```python
from build123d import *

# Parameters (mm, degrees)
F0_W     = 152.4
F0_H     = 101.6
F1_DEPTH = 7.62
F2_T     = -2.54
F3_R     = 5.08


with BuildPart() as f1:
    # F0 (on Front) → F1 (new body)
    with BuildSketch(Plane.XZ):
        Rectangle(F0_W, F0_H)
    extrude(amount=F1_DEPTH)

    # F2
    f2_openings = [f1.faces().sort_by_distance(p)[0] for p in [
        (0, -7.62, 0),
    ]]
    offset(amount=F2_T, openings=f2_openings)

    # F3
    f3_edges = [f1.edges().sort_by_distance(p)[0] for p in [
        (-73.66, -5.08, 48.26),
        (-73.66, -5.08, -48.26),
        (73.66, -5.08, 48.26),
        (73.66, -5.08, -48.26),
    ]]
    fillet(f3_edges, radius=F3_R)


solid = f1.part
```
Read the model definition and answer for the solid it produces. Units are mm, in the model's axes. A direction names the side the tool comes from. Coordinates: 2 decimals unless noted, no trailing zeros. Loops run counter-clockwise (first coordinate to the right, second up) from the corner with the lowest first, then second, coordinate; pieces in that order, holes last.
(1) The part is cut by section B-B (x = 49). Determine the outline of the cut face in (y, z), and give its area (3 significant figures).
Solution:
outline: (-7.62, -50.8) - (0, -50.8) - (0, 50.8) - (-7.62, 50.8) - (-7.62, 48.26) - (-2.54, 48.26) - (-2.54, -48.26) - (-7.62, -48.26) - close
area: 284 mm2
(2) The part is cut by section C-C (z = 37.5). Determine the outline of the cut face in (x, y), and give its area (3 significant figures).
Solution:
outline: (-76.2, -7.62) - (-73.66, -7.62) - (-73.66, -2.54) - (73.66, -2.54) - (73.66, -7.62) - (76.2, -7.62) - (76.2, 0) - (-76.2, 0) - close
area: 413 mm2
(3) Consider line 1 along X through (y, z) = (-3, -43); line 2 along Z through (x, y) = (-18.5, -3.25); line 3 along Y through (x, z) = (-67, -34.5). Determine where each line is inside the solid, lowest interval first.
Solution:
line 1: x = -76.2 to -73.66, 73.66 to 76.2
line 2: z = -50.8 to -48.26, 48.26 to 50.8
line 3: y = -2.54 to 0
(4) The part is cut by section A-A (y = -5.25). Determine the outline of the cut face in (x, z).
Solution:
outline: (-76.2, -50.8) - (76.2, -50.8) - (76.2, 50.8) - (-76.2, 50.8) - close; hole (-73.66, -43.18) arc R5.08 ccw to (-68.58, -48.26) - (68.58, -48.26) arc R5.08 ccw to (73.66, -43.18) - (73.66, 43.18) arc R5.08 ccw to (68.58, 48.26) - (-68.58, 48.26) arc R5.08 ccw to (-73.66, 43.18) - close
(5) A flat-ended cylindrical pin translates along its axis: pin 1 Ø1 at (x, z) = (36, -23) entering from -Y. Find the tip coordinate at first contact, or state that the pin passes through.
Solution:
pin 1: stops at y = -2.54
(6) The mould has two halves that part along X. Classify faces 1 (the face through (-76.2, -4, -1)), 2 (the face through (-1, -5, 48.26)), 3 (the face through (-1, -4, 50.8)), 4 (the face through (76.2, -4, -1)): released by +X, released by -X, zero draft, split by the parting line, or undercut.
Solution:
face 1: released by -X
face 2: undercut
face 3: zero draft
face 4: released by +X
(7) A tool of negligible diameter and unlimited length cuts with its end or side. For faces 5 (the face through (73.66, -5, -1)), 6 (the face through (-1, -4, -50.8)), from which of +Z, -Z, +X, -X, +Y, -Y can it reach the whole face along a straight path? Write none if from no direction.
Solution:
face 5: -Y
face 6: -Z, +X, -X, +Y, -Y
